For this review, use the dimensioned drawing (mm, ordinates from the lowest corner) and the shaded views. A direction names the side the tool comes from. Coordinates: 2 decimals unless noted, no trailing zeros. Write each loop counter-clockwise with the first axis right and the second up, starting at its lowest first coordinate (ties: lowest second). Pieces come first, ordered by that corner, then holes. Notation, with made-up numbers: (55.25, 68.5) - (69.25, 68.5) arc R20 ccw to (69.25, 104.5) - close; hole circle Ø4 at (37, 83.5). An arc over 180 degrees is marked (long way). Answer as a JSON object with one key per item and string values.
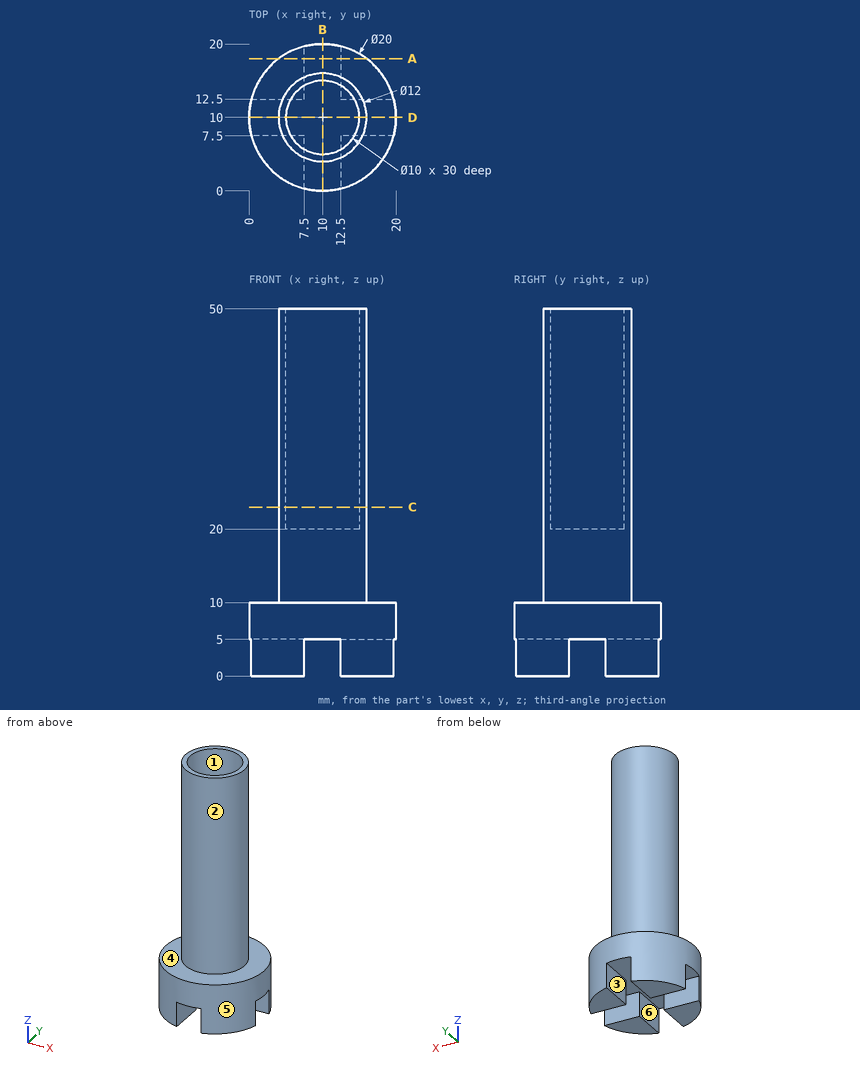
(1) For pin 1 (2.5 mm diameter, centred on y = 16, z = 3.5, fed in from +X); pin 2 (12 mm diameter, centred on x = 15, z = 30, fed in from -Y); pin 3 (5.5 mm diameter, centred on x = 2, z = 2, fed in from +Y), all flat-tipped, find the tip position at first contact; note any pin that passes through.
Solved:
{"pin 1": "stops at x = 18.8", "pin 2": "stops at y = 4", "pin 3": "stops at y = 18.51"}
(2) Take a section at C-C, the plane z = 23. Write out the cut boundary in (x, y).
Solved:
{"outline": "circle Ø12 at (10, 10); hole circle Ø10 at (10, 10)"}
(3) Take a section at B-B, the plane x = 10. Write out the cut boundary in (y, z), and give its area (3 significant figures).
Solved:
{"outline": "(0, 5) - (20, 5) - (20, 10) - (16, 10) - (16, 50) - (15, 50) - (15, 20) - (5, 20) - (5, 50) - (4, 50) - (4, 10) - (0, 10) - close", "area": "280 mm^2"}
(4) Take a section at A-A, the plane y = 18. Write out the cut boundary in (x, z), and give its area (3 significant figures).
Solved:
{"outline": "(4, 0) - (7.5, 0) - (7.5, 5) - (12.5, 5) - (12.5, 0) - (16, 0) - (16, 10) - (4, 10) - close", "area": "95.0 mm^2"}
(5) Tool access review of the marked faces 4, 5 and 6: name each direction out of +Z, -Z, +X, -X, +Y, -Y from which nothing blocks a thin tool from reaching the whole face with its end or side.
Solved:
{"face 4": "+Z", "face 5": "+Z, -Z", "face 6": "-Z, +Y, -Y"}
(6) To check wall thickness, follow line 1 (Y direction, x = 10, z = 27.25); line 2 (Z direction, x = 14, y = 1.25); line 3 (Y direction, x = 14, z = 47). State the ranges of each line that lie inside material, in increasing order. Write a range as from..to.
Solved:
{"line 1": "y = 4..5, 15..16", "line 2": "z = 0..10", "line 3": "y = 5.53..7, 13..14.47"}
(7) The part is to be moulded in two halves that separate along Y. For the marked faces 1, 2 and 3, say which applies: pulls with the +Y half, pulls with the -Y half, needs draft (parallel to the pull), parting line crosses it, or undercut.
Solved:
{"face 1": "undercut", "face 2": "parting line crosses it", "face 3": "needs draft"}
